Check sheet for the modelled part. Datum: model origin and axes. Units: mm. Face numbers are marked on the shaded views. A direction names the side the tool comes from. Round coordinates to 2 decimals unless told otherwise and drop trailing zeros. Write each loop counter-clockwise with the first axis right and the second up, starting at its lowest first coordinate (ties: lowest second). Pieces come first, ordered by that corner, then holes. Notation, with made-up numbers: M 56,75 L 108,75 A15 ccw 108,87 Z; hole C -26,16 d3. An arc over 180 degrees is marked long. Answer in a Markdown table with one row per item.
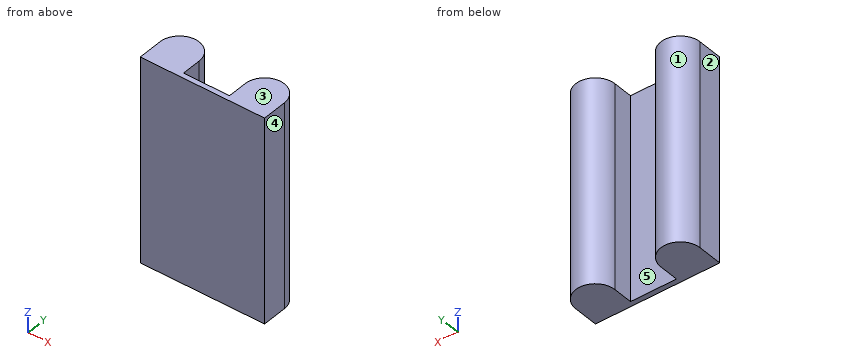
```python
from build123d import *

# Parameters (mm, degrees)
SKETCH1_W           = 73
SKETCH1_H           = 3
BOSS_EXTRUDE1_DEPTH = 120


with BuildPart() as part:
    # Sketch1 → Boss-Extrude1 (new body)
    with BuildSketch(Plane.XY):
        with BuildLine():
            ThreePointArc((11.5, 0), (0, 11.5), (-11.5, 0))
            Line((-11.5, 0), (11.5, 0))
        make_face()
        with BuildLine():
            Line((11.5, 0), (-11.5, 0))
            ThreePointArc((-11.5, 0), (-8.131727984, -8.131727984), (0, -11.5))
            ThreePointArc((0, -11.5), (8.131727984, -8.131727984), (11.5, 0))
        make_face()
        with BuildLine():
            ThreePointArc((11.5, 0), (0, 11.5), (-11.5, 0))
            Line((-11.5, 0), (11.5, 0))
        make_face()
        with BuildLine():
            Line((11.5, 0), (-11.5, 0))
            ThreePointArc((-11.5, 0), (-8.131727984, -8.131727984), (0, -11.5))
            ThreePointArc((0, -11.5), (8.131727984, -8.131727984), (11.5, 0))
        make_face()
        with BuildLine():
            Line((11.5, -11.5), (11.5, 0))
            ThreePointArc((11.5, 0), (8.131727984, -8.131727984), (0, -11.5))
            Line((0, -11.5), (11.5, -11.5))
        make_face()
        with BuildLine():
            ThreePointArc((0, -11.5), (-8.131727984, -8.131727984), (-11.5, 0))
            Line((-11.5, 0), (-11.5, -11.5))
            Line((-11.5, -11.5), (0, -11.5))
        make_face()
        with BuildLine():
            ThreePointArc((50, -11.5), (41.868272016, -8.131727984), (38.5, 0))
            Line((38.5, 0), (38.5, -11.5))
            Line((38.5, -11.5), (50, -11.5))
        make_face()
        with BuildLine():
            ThreePointArc((61.5, 0), (50, 11.5), (38.5, 0))
            Line((38.5, 0), (61.5, 0))
        make_face()
        with BuildLine():
            Line((61.5, 0), (38.5, 0))
            ThreePointArc((38.5, 0), (41.868272016, -8.131727984), (50, -11.5))
            ThreePointArc((50, -11.5), (58.131727984, -8.131727984), (61.5, 0))
        make_face()
        with BuildLine():
            ThreePointArc((61.5, 0), (50, 11.5), (38.5, 0))
            Line((38.5, 0), (61.5, 0))
        make_face()
        with BuildLine():
            Line((61.5, 0), (38.5, 0))
            ThreePointArc((38.5, 0), (41.868272016, -8.131727984), (50, -11.5))
            ThreePointArc((50, -11.5), (58.131727984, -8.131727984), (61.5, 0))
        make_face()
        with BuildLine():
            Line((61.5, -11.5), (61.5, 0))
            ThreePointArc((61.5, 0), (58.131727984, -8.131727984), (50, -11.5))
            Line((50, -11.5), (61.5, -11.5))
        make_face()
        with Locations((25, -13)):
            Rectangle(SKETCH1_W, SKETCH1_H)
    extrude(amount=BOSS_EXTRUDE1_DEPTH)


solid = part.part
```
1. Section check A-A, the plane y = -1.75. Record the cut outline in (x, z).
Found:
| item | result |
|---|---|
| outline | M -11.5,0 L 11.5,0 L 11.5,120 L -11.5,120 Z; M 38.5,0 L 61.5,0 L 61.5,120 L 38.5,120 Z |
2. Section check D-D, the plane x = 47. Record the cut outline in (y, z).
Found:
| item | result |
|---|---|
| outline | M -14.5,0 L 11.1,0 L 11.1,120 L -14.5,120 Z |
3. Draft check along X on the marked faces 1, 2 and 3. Enter one of: +X half, -X half, draft (parallel to the pull), parting line (faces both ways), or undercut.
Found:
| item | result |
|---|---|
| face 1 | undercut |
| face 2 | -X half |
| face 3 | draft |
4. Section check B-B, the plane z = 54.5. Record the cut outline in (x, y).
Found:
| item | result |
|---|---|
| outline | M -11.5,-14.5 L 61.5,-14.5 L 61.5,0 A11.5 ccw 38.5,0 L 38.5,-11.5 L 11.5,-11.5 L 11.5,0 A11.5 ccw -11.5,0 Z |
5. Section check C-C, the plane x = 25. Record the cut outline in (y, z).
Found:
| item | result |
|---|---|
| outline | M -14.5,0 L -11.5,0 L -11.5,120 L -14.5,120 Z |
6. Scan lines: L1, parallel to X at y = -2.5, z = 85; L2, parallel to Y at x = 33, z = 102; L3, parallel to X at y = 5.5, z = 47.5. Record each from-to range of solid material in increasing order.
Found:
| item | result |
|---|---|
| L1 | x = -11.5 to 11.5, 38.5 to 61.5 |
| L2 | y = -14.5 to -11.5 |
| L3 | x = -10.1 to 10.1, 39.9 to 60.1 |
7. Access from +Z, -Z, +X, -X, +Y, -Y to the whole of each face (thin tool, end or side, straight path). Record for the marked faces 4 and 5.
Found:
| item | result |
|---|---|
| face 4 | +Z, -Z, +X, +Y, -Y |
| face 5 | +Z, -Z, +Y |
8. Go/stop test with flat-tipped pins: pin 1 (3 mm diameter, centred on y = 7, z = 78, fed in from -X); pin 2 (13.5 mm diameter, centred on x = 26.5, z = 32, fed in from +Y). Record where each tip stops, or that it passes through.
Found:
| item | result |
|---|---|
| pin 1 | stops at x = -10.1 |
| pin 2 | stops at y = -11.5 |
